Verification items for the finished model (mm, model axes). Face numbers are marked on the shaded views. Round coordinates to 2 decimals unless told otherwise and drop trailing zeros. Write each loop counter-clockwise with the first axis right and the second up, starting at its lowest first coordinate (ties: lowest second). Pieces come first, ordered by that corner, then holes.
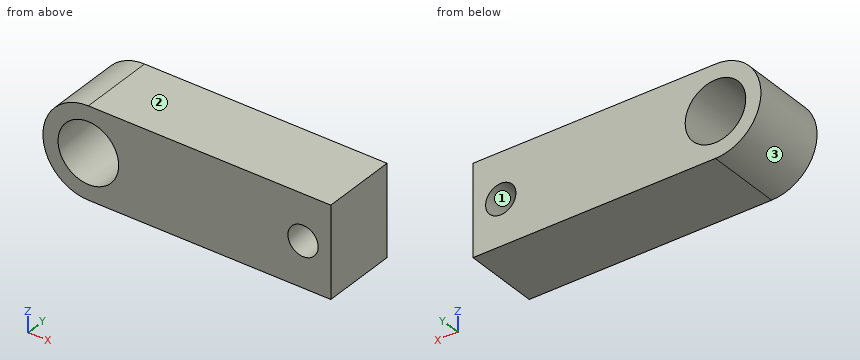
from build123d import *

# Parameters (mm, degrees)
EXTRUDE_1_DEPTH     = 5
SKETCH_3_R          = 2
CUT_EXTRUDE_1_DEPTH = 5
SKETCH_4_R          = 1
CUT_EXTRUDE_2_DEPTH = 5


with BuildPart() as part:
    # 草图2 → 凸台-拉伸1 (new body)
    with BuildSketch(Plane(origin=(0, 0, 0), x_dir=(1, 0, 0), z_dir=(0, 1, 0))):
        with BuildLine():
            Line((0, 3), (16, 3))
            Line((16, 3), (16, -3))
            Line((16, -3), (0, -3))
            ThreePointArc((0, -3), (-3, 0), (0, 3))
        make_face()
    extrude(amount=EXTRUDE_1_DEPTH)

    # 草图3 → 切除-拉伸1 (cut)
    with BuildSketch(Plane(origin=(0, 5, 0), x_dir=(1, 0, 0), z_dir=(0, 1, 0))):
        with Locations(Location((0, 0, 0), (0, 0, 270))):
            Circle(SKETCH_3_R)
    extrude(amount=-CUT_EXTRUDE_1_DEPTH, mode=Mode.SUBTRACT)

    # 草图4 → 切除-拉伸2 (cut)
    with BuildSketch(Plane(origin=(0, 5, 0), x_dir=(1, 0, 0), z_dir=(0, 1, 0))):
        with Locations(Location((14.167639534, 0, 0), (0, 0, 270))):
            Circle(SKETCH_4_R)
    extrude(amount=-CUT_EXTRUDE_2_DEPTH, mode=Mode.SUBTRACT)


solid = part.part
Q1. Material ranges on line 1 along X through (y, z) = (2.65, 0); line 2 along X through (y, z) = (4.15, 0.3); line 3 along X through (y, z) = (0.4, -1.6), recorded low to high.
Recorded:
line 1: x = -3 to -2, 2 to 13.17, 15.17 to 16
line 2: x = -2.98 to -1.98, 1.98 to 13.21, 15.12 to 16
line 3: x = -2.54 to -1.2, 1.2 to 16
Q2. Release check for a two-part mould opening along X. For the marked faces 1, 2 and 3 record: released by +X, released by -X, zero draft, split by the parting line, or undercut.
Recorded:
face 1: undercut
face 2: zero draft
face 3: released by -X
Q3. Sectioned sample at B-B (x = 13.75). Enter the section's corners in (y, z).
Recorded:
outline: (0, -3) - (5, -3) - (5, -0.91) - (0, -0.91) - close; (0, 0.91) - (5, 0.91) - (5, 3) - (0, 3) - close
Q4. Sectioned sample at A-A (z = 0). Enter the section's corners in (x, y).
Recorded:
outline: (-3, 0) - (-2, 0) - (-2, 5) - (-3, 5) - close; (2, 0) - (13.17, 0) - (13.17, 5) - (2, 5) - close; (15.17, 0) - (16, 0) - (16, 5) - (15.17, 5) - close
Q5. Sectioned sample at D-D (z = -0.8). Enter the section's corners in (x, y), plus the area to 3 significant figures.
Recorded:
outline: (-2.89, 0) - (-1.83, 0) - (-1.83, 5) - (-2.89, 5) - close; (1.83, 0) - (13.57, 0) - (13.57, 5) - (1.83, 5) - close; (14.77, 0) - (16, 0) - (16, 5) - (14.77, 5) - close
area: 70.1 mm2
Q6. Sectioned sample at C-C (y = 4.1). Enter the section's corners in (x, z).
Recorded:
outline: (0, -3) - (16, -3) - (16, 3) - (0, 3) arc R3 ccw to start; hole circle Ø4 at (0, 0); hole circle Ø2 at (14.17, 0)
